The listing builds one solid part. Answer for the finished solid, in the listing's coordinates (mm). Coordinates: 2 decimals unless noted, no trailing zeros. Order: outer loops, then holes, each group sorted by start corner. A loop starts at its lowest first (then second) coordinate and runs counter-clockwise, first axis right, second up. Notation, with made-up numbers: (5.25, 1) - (58.25, 1) arc R21 ccw to (58.25, 17) - close; hole circle Ø2 at (-15, -33.5). An arc over 180 degrees is marked (long way). Use one line per item in the form item = value. Start each with the question number.
Item 1: The mould has two halves that part along Y. Classify faces 1 (the cylindrical face through (-0.13, 378.28, -16.19)), 2 (the cylindrical face through (0.1, -50.8, 0.2)), 3 (the cylindrical face through (-0.13, -1.72, -7.75)): released by +Y, released by -Y, zero draft, split by the parting line, or undercut.
Item 2: Section B-B, the plane z = 0 is taken. Write down the section's boundary in (x, y) (1 decimal).
Item 3: Consider line 1 along Y through (x, z) = (0, 10.25); line 2 along Y through (x, z) = (0.25, 6); line 3 along Y through (x, z) = (-0.75, -2.5). Determine where each line is inside the solid, lowest interval first. Write a range as [from, to].
Item 4: Each of these flat-tipped pins is pushed along its axis until it touches: pin 1 Ø14.5 at (y, z) = (0, 0) entering from -X; pin 2 Ø10 at (x, z) = (4, -12) entering from -Y; pin 3 Ø1 at (x, y) = (-0.5, 263) entering from +Z. Where does it stop, or does it pass through?
from build123d import *

# Parameters (mm, degrees)
F0_R     = 7.9375
F1_DEPTH = 9.525
F2_R     = 1.5875
F3_DEPTH = 25.4
F4_R     = 9.525
F5_R     = 3.175


with BuildPart() as f1:
    # F0 (on Right) → F1 (new body, symmetric)
    with BuildSketch(Plane.YZ):
        with BuildLine():
            Line((381, -19.05), (381, 19.05))
            Line((381, 19.05), (-47.09286, 19.05))
            ThreePointArc((-47.09286, 19.05), (-50.8, 0), (-47.09286, -19.05))
            Line((-47.09286, -19.05), (381, -19.05))
        make_face()
        Circle(F0_R, mode=Mode.SUBTRACT)
    extrude(amount=F1_DEPTH, both=True)

    # F2 (on face) → F3 (cut)
    with BuildSketch(Plane.XY.offset(19.05)):
        with Locations((0, 346.075)):
            Circle(F2_R)
        with Locations((0, 263.525)):
            Circle(F2_R)
    extrude(amount=-F3_DEPTH, mode=Mode.SUBTRACT)

    # F4
    f4_edges = [f1.edges().sort_by_distance(p)[0] for p in [
        (0, 381, -19.05),
    ]]
    fillet(f4_edges, radius=F4_R)

    # F5
    f5_edges = [f1.edges().sort_by_distance(p)[0] for p in [
        (0, 381, 19.05),
        (0, -47.09286, -19.05),
        (0, -47.09286, 19.05),
    ]]
    fillet(f5_edges, radius=F5_R)


solid = f1.part
Response:
q1.face_1 = released by +Y
q1.face_2 = released by -Y
q1.face_3 = undercut
q2.outline = (-9.5, -50.8) - (9.5, -50.8) - (9.5, -7.9) - (-9.5, -7.9) - close; (-9.5, 7.9) - (9.5, 7.9) - (9.5, 381) - (-9.5, 381) - close; hole circle Ø3.2 at (0, 263.5); hole circle Ø3.2 at (0, 346.1)
q3.line_1 = [-49.76, 261.94], [265.11, 344.49], [347.66, 381]
q3.line_2 = [-50.44, -5.2], [5.2, 261.96], [265.09, 344.51], [347.64, 381]
q3.line_3 = [-50.74, -7.53], [7.53, 262.13], [264.92, 344.68], [347.47, 381]
q4.pin_1 = through
q4.pin_2 = -50.32
q4.pin_3 = -6.35
